Autodesk Inventor part; units mm, degrees
ref_plane "YZ Plane" through (0, 0, 0) normal (1, 0, 0) x (0, 1, 0)
ref_plane "XZ Plane" through (0, 0, 0) normal (0, 1, 0) x (-1, 0, 0)
ref_plane "XY Plane" through (0, 0, 0) normal (0, 0, 1) x (1, 0, 0)
sketch "Skizze1" plane through (0, 0, 0) normal (0, 1, 0) x (-1, 0, 0)
  line L0 (0, 3.5) -> (14, 3.5)
  line L1 (14, 3.5) -> (14, -3.5)
  line L2 (14, -3.5) -> (0, -3.5)
  line L3 (0, -3.5) -> (0, 3.5)
  point P0 (0, 0)
  point P1 (0, 0)
  dimension "d0" = 7
  dimension "d1" = 14
extrude "Extrusion1" add sketch "Skizze1" along normal blind 8
fillet "Rundung1" radius 3.5 2 edges at (-14, 4, -3.5) (-14, 4, 3.5)
sketch "Skizze2" plane through (0, 8, 0) normal (0, 1, 0) x (1, 0, 0)
  arc A0 (-10.5, 3.5) -> (-10.5, -3.5) centre (-10.5, 0) ccw
  point P0 (0, 0)
hole "Bohrung1" at (-10.5, 8, 0) direction (0, -1, 0) diameter 2 depth 8
sketch "Skizze3" plane through (0, 0, -3.5) normal (0, 0, -1) x (-1, 0, 0)
  line L0 (7.5, 6) -> (16, 6)
  line L1 (16, 6) -> (16, 2)
  line L2 (16, 2) -> (7.5, 2)
  line L3 (7.5, 2) -> (7.5, 6)
  line L4 (14, 0) -> (14, 8)
  line L5 (0, 0) -> (0, 8)
  point P0 (7.5, 4)
  point P1 (0, 4)
  point P2 (11.75, 2)
  point P3 (16, 4)
  dimension "d12" = 6.5
  dimension "d13" = 4
  dimension "d14" = 2
extrude "Extrusion2" cut sketch "Skizze3" against normal up to surface (7 mm away)
sketch "Skizze4" plane through (0, 0, 3.5) normal (1, 0, 0) x (0, 0, -1)
  circle A0 centre (3.5, 4) radius 1.5
  line L0 (7, 0) -> (7, 8)
  line L1 (0, 0) -> (7, 0)
  point P0 (3.5, 0)
  point P1 (7, 4)
  point P2 (3.5, 0)
  dimension "d17" = 3
extrude "Extrusion3" add sketch "Skizze4" along normal blind 5
thread "Gewinde1"
properties part number "25"
For this review, take the finished solid that the model builds, in its own axes (mm). A direction names the side the tool comes from. Round coordinates to 2 decimals unless told otherwise and drop trailing zeros. Loops run counter-clockwise (first coordinate to the right, second up) from the corner with the lowest first, then second, coordinate; pieces in that order, holes last. Notation, with made-up numbers: (-9, 75.25) - (15, 75.25) arc R16 ccw to (15, 86.25) - close; hole circle Ø6 at (-32, 12.25). An arc over 180 degrees is marked (long way). Use one line per item in the form item = value.
1) We need section B-B on z = -0.25. Write out the cut boundary in (x, y).
Solutions:
outline = (-13.99, 0) - (-11.47, 0) - (-11.47, 2) - (-13.99, 2) - close; (-13.99, 6) - (-11.47, 6) - (-11.47, 8) - (-13.99, 8) - close; (-9.53, 0) - (0, 0) - (0, 2.52) - (5, 2.52) - (5, 5.48) - (0, 5.48) - (0, 8) - (-9.53, 8) - (-9.53, 6) - (-7.5, 6) - (-7.5, 2) - (-9.53, 2) - close
2) Tool access review of faces 5 (the face through (-7.5, 4, 0)), 6 (the face through (-11.49, 6.99, -0.13)), 7 (the face through (0, 4, -2)): name each direction out of +Z, -Z, +X, -X, +Y, -Y from which nothing blocks a thin tool from reaching the whole face with its end or side.
Solutions:
face_5 = +Z, -Z, -X
face_6 = +Y, -Y
face_7 = +X
3) We need section D-D on z = 2.25. Write out the cut boundary in (x, y).
Solutions:
outline = (-13.18, 0) - (0, 0) - (0, 8) - (-13.18, 8) - (-13.18, 6) - (-7.5, 6) - (-7.5, 2) - (-13.18, 2) - close
4) Mouldability with a two-part tool opening along Z and no side actions: class faces 1 (the face through (-11.43, 6, 0.73)), 2 (the face through (-11.49, 0.99, -0.13)), 3 (the face through (-4, 4, 3.5)), 4 (the face through (-4, 4, -3.5)) as pulls with the +Z half, pulls with the -Z half, needs draft (parallel to the pull), parting line crosses it, or undercut.
Solutions:
face_1 = needs draft
face_2 = undercut
face_3 = pulls with the +Z half
face_4 = pulls with the -Z half
5) We need section A-A on y = 4. Write out the cut boundary in (x, z).
Solutions:
outline = (-7.5, -3.5) - (0, -3.5) - (0, -1.5) - (5, -1.5) - (5, 1.5) - (0, 1.5) - (0, 3.5) - (-7.5, 3.5) - close
6) Clearance check with flat-ended pins moving along their axes: P1, Ø1, axis at y = 1, z = -1, coming from the +X side; P2, Ø2, axis at x = -9, z = 1, coming from the -Y side. State where each tip first meets the part, or that it passes through.
Solutions:
P1 = 0
P2 = 0
7) Wall thickness on probe 1 along X at (y, z) = (1, 0); probe 2 along Y at (x, z) = (-11.25, -1.25); probe 3 along Z at (x, y) = (-10.5, 1.35): over which ranges is each line inside the solid? List them lowest first.
Solutions:
probe_1 = -14 to -11.5, -9.5 to 0
probe_2 = 0 to 2, 6 to 8
probe_3 = -3.5 to -1, 1 to 3.5
